Check sheet for the modelled part. Datum: model origin and axes. Units: mm. A direction names the side the tool comes from. Round coordinates to 2 decimals unless told otherwise and drop trailing zeros. Write each loop counter-clockwise with the first axis right and the second up, starting at its lowest first coordinate (ties: lowest second). Pieces come first, ordered by that corner, then holes.
Item 1: Tool access check on faces 1 (the flat face through (0, 36, 172)), 2 (the flat face through (10, 20, 172)). Record the directions out of +Z, -Z, +X, -X, +Y, -Y that give a thin tool (end or side, any length) a straight path to the whole face; none if there is none.
Item 2: Release check for a two-part mould opening along Y. For faces 3 (the flat face through (0, 4, 172)), 4 (the flat face through (-6, 0, 172)), 5 (the flat face through (10, 36, 172)), 6 (the flat face through (3, 30, 172)) record: +Y half, -Y half, draft (parallel to the pull), parting line (faces both ways), or undercut.
Item 3: Material ranges on line 1 (Y direction, x = -5.75, z = 156); line 2 (Y direction, x = 8.5, z = 327); line 3 (Y direction, x = 3.5, z = 284.5), recorded low to high.
Item 4: Cross-section at A-A on x = 0. Enter the section's corners in (y, z).
from build123d import *

# Parameters (mm, degrees)
EXTRUDE_1_DEPTH = 348
FILLET_1_R      = 0.5


with BuildPart() as part:
    # 草圖1 → 填料-伸長1 (new body)
    with BuildSketch(Plane.XY):
        Polygon((-4.5, 4), (4.5, 4), (4.5, 1), (3, 1), (3, 0), (10, 0), (10, 7), (8, 7), (8, 5.5), (3, 5.5), (3, 14.5), (8, 14.5), (8, 13), (10, 13), (10, 27), (8, 27), (8, 25.5), (3, 25.5), (3, 34.5), (8, 34.5), (8, 33), (10, 33), (10, 40), (3, 40), (3, 39), (4.5, 39), (4.5, 36), (-4.5, 36), (-4.5, 39), (-3, 39), (-3, 40), (-10, 40), (-10, 33), (-8, 33), (-8, 34.5), (-3, 34.5), (-3, 25.5), (-8, 25.5), (-8, 27), (-10, 27), (-10, 13), (-8, 13), (-8, 14.5), (-3, 14.5), (-3, 5.5), (-8, 5.5), (-8, 7), (-10, 7), (-10, 0), (-3, 0), (-3, 1), (-4.5, 1), align=None)
    extrude(amount=EXTRUDE_1_DEPTH)

    # 圓角1
    fillet_1_edges = [part.edges().sort_by_distance(p)[0] for p in [
        (-10, 0, 174),
        (-10, 7, 174),
        (-10, 13, 174),
        (-10, 27, 174),
        (-10, 33, 174),
        (-10, 40, 174),
        (10, 40, 174),
        (10, 33, 174),
        (10, 27, 174),
        (10, 13, 174),
        (10, 7, 174),
        (10, 0, 174),
    ]]
    fillet(fillet_1_edges, radius=FILLET_1_R)


solid = part.part
Response values:
1. face 1: +Z, -Z
1. face 2: +Z, -Z, +X, +Y, -Y
2. face 3: undercut
2. face 4: -Y half
2. face 5: draft
2. face 6: undercut
3. line 1: y = 0 to 5.5, 14.5 to 25.5, 34.5 to 40
3. line 2: y = 0 to 7, 13 to 27, 33 to 40
3. line 3: y = 0 to 1, 4 to 5.5, 14.5 to 25.5, 34.5 to 36, 39 to 40
4. outline: (4, 0) - (36, 0) - (36, 348) - (4, 348) - close
